Part model, mm, in its own coordinate system. Face numbers are marked on the shaded views. A direction names the side the tool comes from. Give positions to 0.01 mm unless a question says otherwise; leave off trailing zeros. Write each loop counter-clockwise with the first axis right and the second up, starting at its lowest first coordinate (ties: lowest second). Pieces come first, ordered by that corner, then holes.
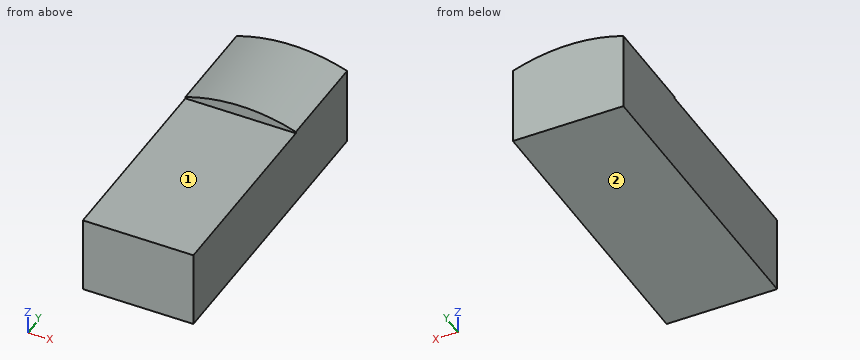
from build123d import *

# Parameters (mm, degrees)
BOX001_W            = 10
BOX001_H            = 18
BOX001_DEPTH        = 10
BOX_W               = 10
BOX_H               = 27
BOX_DEPTH           = 8
CYLINDER_R          = 15
CYLINDER_DEPTH      = 40
CYLINDER_ROLL_ANGLE = 90


with BuildPart() as flat_top:
    # Box001 → Box001 (new body)
    with BuildSketch(Plane.XY.offset(7)):
        with Locations((5, 9)):
            Rectangle(BOX001_W, BOX001_H)
    extrude(amount=BOX001_DEPTH)


with BuildPart() as pin:
    # Box → Box (new body)
    with BuildSketch(Plane.XY):
        with Locations((5, 13.5)):
            Rectangle(BOX_W, BOX_H)
    extrude(amount=BOX_DEPTH)


with BuildPart() as cut:
    # Cylinder → Cylinder (new body)
    with BuildSketch(Plane.XY):
        Circle(CYLINDER_R)
    extrude(amount=CYLINDER_DEPTH)


with BuildPart() as cut_1:
    # Cylinder roll: moved
    add(cut.part.rotate(Axis((0, 0, 0), (1, 0, 0)), CYLINDER_ROLL_ANGLE))


with BuildPart() as cut_2:
    # Cylinder placement: moved
    add(cut_1.part.moved(Location((5, 35, -7))))

    # Common: intersect pin
    add(pin.part, mode=Mode.INTERSECT)

    # Cut: cut flat_top
    add(flat_top.part, mode=Mode.SUBTRACT)


with BuildPart() as cut_3:
    # Cut placement: moved
    add(cut_2.part.moved(Location((0, 11, 0))))


solid = cut_3.part
1) Saw through at B-B (x = 1). Write the cut outline in (y, z), and give its area (3 significant figures).
Check result:
outline: (11, 0) - (38, 0) - (38, 7.46) - (29, 7.46) - (29, 7) - (11, 7) - close
area: 193 mm2
2) Flat gauge pins, fed straight in: P1, Ø1.5, axis at x = 5, y = 20, coming from the +Z side; P2, Ø2, axis at x = 2, y = 29, coming from the +Z side; P3, Ø3, axis at y = 26, z = 4.5, coming from the -X side. Where does each tip first touch, or does it go through?
Check result:
P1: stops at z = 7
P2: stops at z = 7.87
P3: stops at x = 0
3) Drill centre lines: L1, parallel to Z at x = 4.25, y = 16; L2, parallel to Y at x = 7.25, z = 7.5; L3, parallel to Z at x = 3, y = 32.5. Where is each one in solid material? Low to high.
Check result:
L1: z = 0 to 7
L2: y = 29 to 38
L3: z = 0 to 7.87
4) Saw through at D-D (y = 34.5). Write the cut outline in (x, z).
Check result:
outline: (0, 0) - (10, 0) - (10, 7.14) arc R15 ccw to (0, 7.14) - close
5) Saw through at A-A (y = 20.5). Write the cut outline in (x, z), and give its area (3 significant figures).
Check result:
outline: (0, 0) - (10, 0) - (10, 7) - (0, 7) - close
area: 70.0 mm2
6) Saw through at C-C (x = 6.25). Write the cut outline in (y, z).
Check result:
outline: (11, 0) - (38, 0) - (38, 7.95) - (29, 7.95) - (29, 7) - (11, 7) - close
7) 3-axis set-ups, long thin cutter, end or side, ignore diameter. For the marked faces 1 and 2: which of +Z, -Z, +X, -X, +Y, -Y reach the whole face in a straight line?
Check result:
face 1: +Z, +X, -X, -Y
face 2: -Z, +X, -X, +Y, -Y
